```python
from build123d import *

# Parameters (mm, degrees)
SKETCH1_R           = 6.35
SKETCH1_R_2         = 3.175
BOSS_EXTRUDE1_DEPTH = 3.175
SKETCH1_3_R         = 6.35
BOSS_EXTRUDE2_DEPTH = 4.7625
FILLET1_R           = 6.35
SKETCH4_W           = 50.8
SKETCH4_H           = 4.7625
BOSS_EXTRUDE3_DEPTH = 40
SKETCH5_W           = 50.8
SKETCH5_H           = 3.175
BOSS_EXTRUDE4_DEPTH = 88.9
FILLET2_R           = 3.175
SKETCH11_W          = 25.527
SKETCH11_H          = 76.327
CUT_EXTRUDE2_DEPTH  = 125.625465933
SKETCH12_W          = 2.369732381
SKETCH12_H          = 76.327
SKETCH12_W_2        = 2.555200435
BOSS_EXTRUDE5_DEPTH = 1
CUT_EXTRUDE3_DEPTH  = 125.625465933


with BuildPart() as part:
    # Sketch1 → Boss-Extrude1 (new body)
    with BuildSketch(Plane(origin=(0, 0, 0), x_dir=(1, 0, 0), z_dir=(0, 1, 0))):
        with Locations(Location((0, 0, 0), (0, 0, 270))):
            Circle(SKETCH1_R)
        with Locations(Location((0, 0, 0), (0, 0, 270))):
            Circle(SKETCH1_R_2, mode=Mode.SUBTRACT)
    extrude(amount=BOSS_EXTRUDE1_DEPTH)

    # Sketch1_3 → Boss-Extrude2 (add)
    with BuildSketch(Plane(origin=(0, 0, 0), x_dir=(1, 0, 0), z_dir=(0, 1, 0))):
        Polygon((-12.7, -9.525), (-12.7, 0), (-12.7, 22.232248258), (12.7, 22.232248258), (12.7, 0), (12.7, -9.525), align=None)
        with Locations(Location((0, 0, 0), (0, 0, 90))):
            Circle(SKETCH1_3_R, mode=Mode.SUBTRACT)
    extrude(amount=BOSS_EXTRUDE2_DEPTH)

    # Mirror1: part across plane


with BuildPart() as part_1:
    add(part.part)
    add(part.part.mirror(Plane(origin=(12.7, 0, 0), x_dir=(0, 0, 1), z_dir=(1, 0, 0))))

    # Fillet1
    fillet1_edges = [part_1.edges().sort_by_distance(p)[0] for p in [
        (38.1, 2.38125, 9.525),
        (-12.7, 2.38125, 9.525),
    ]]
    fillet(fillet1_edges, radius=FILLET1_R)

    # Sketch4 → Boss-Extrude3 (add)
    with BuildSketch(Plane.XZ):
        with Locations((12.7, -19.850998258)):
            Rectangle(SKETCH4_W, SKETCH4_H)
    extrude(amount=BOSS_EXTRUDE3_DEPTH)

    # Sketch5 → Boss-Extrude4 (add)
    with BuildSketch(Plane(origin=(0, 0, -22.232248258), x_dir=(-1, 0, 0), z_dir=(0, 0, -1))):
        with Locations((-12.7, -38.4125)):
            Rectangle(SKETCH5_W, SKETCH5_H)
    extrude(amount=BOSS_EXTRUDE4_DEPTH)

    # Fillet2
    fillet2_edges = [part_1.edges().sort_by_distance(p)[0] for p in [
        (38.1, -38.4125, -111.132248258),
        (-12.7, -38.4125, -111.132248258),
    ]]
    fillet(fillet2_edges, radius=FILLET2_R)

    # Sketch11 → Cut-Extrude2 (cut, through all)
    with BuildSketch(Plane(origin=(0, -36.825, 0), x_dir=(1, 0, 0), z_dir=(0, 1, 0))):
        with Locations((12.6365, 60.395748258)):
            Rectangle(SKETCH11_W, SKETCH11_H)
    extrude(amount=-CUT_EXTRUDE2_DEPTH, mode=Mode.SUBTRACT)

    # Sketch12 → Boss-Extrude5 (add)
    with BuildSketch(Plane.XZ.offset(40)):
        with Locations((1.05786619, -60.395748258)):
            Rectangle(SKETCH12_W, SKETCH12_H)
        with Locations((24.122399783, -60.395748258)):
            Rectangle(SKETCH12_W_2, SKETCH12_H)
    extrude(amount=-BOSS_EXTRUDE5_DEPTH)

    # Sketch14 → Cut-Extrude3 (cut, through all)
    with BuildSketch(Plane(origin=(0, -36.825, 0), x_dir=(1, 0, 0), z_dir=(0, 1, 0))):
        with BuildLine():
            Line((0.534999946, 104.782248258), (0.534999946, 111.132248258))
            Line((0.534999946, 111.132248258), (24.664999946, 111.132248258))
            Line((24.664999946, 111.132248258), (24.664999946, 104.782248258))
            ThreePointArc((24.664999946, 104.782248258), (24.201028616, 101.468585813), (22.844799565, 98.409783604))
            Line((22.844799565, 98.409783604), (22.844799565, 98.559248258))
            Line((22.844799565, 98.559248258), (2.242732381, 98.559248258))
            Line((2.242732381, 98.559248258), (2.242732381, 98.594257179))
            ThreePointArc((2.242732381, 98.594257179), (0.96976654, 101.572591591), (0.534999946, 104.782248258))
        make_face()
    extrude(amount=-CUT_EXTRUDE3_DEPTH, mode=Mode.SUBTRACT)


solid = part_1.part
```
Here's how the part is built. I have some questions about the finished solid (model axes, mm). A direction names the side the tool comes from. Give positions to 0.01 mm unless a question says otherwise; leave off trailing zeros. Write each loop counter-clockwise with the first axis right and the second up, starting at its lowest first coordinate (ties: lowest second). Pieces come first, ordered by that corner, then holes. Notation, with made-up numbers: M -28,21 L 22,21 A13 cw 22,38 Z; hole C 36.5,64.25 d11. An arc over 180 degrees is marked long. Put each result on its own line as item: value. Start each with the question number.
Item 1: If we section it at A-A, the plane z = -53: Write out the boundary of the cut face in (x, y) (3 decimals), then the cut area to 3 significant figures.
Item 2: On a 3-axis mill with a long thin cutter (end or side, diameter ignored), from which of +Z, -Z, +X, -X, +Y, -Y can I reach the whole of each face in a straight line? I mean faces 4 (the flat face through (24, -39, -60)), 5 (the cylindrical face through (-10.889, 2.415, 7.615)), 6 (the flat face through (0.535, -38, -108)). Say none if no direction works.
Item 3: If we section it at D-D, the plane y = -20: Write out the boundary of the cut face in (x, z), then the cut area to 3 significant figures.
Item 4: Thinking about a two-plate mould opening in X: for faces 1 (the flat face through (-12.7, -38, -40)), 2 (the flat face through (-7, -36.825, -66)), 3 (the flat face through (-0.127, -38, -60)), which applies, +X half, -X half, draft (parallel to the pull), parting line (faces both ways), or undercut?
Item 5: I need wall thicknesses on L1, parallel to X at y = 2.35, z = 0 (3 decimals); L2, parallel to Z at x = 25.4, y = 1.15 (3 decimals); L3, parallel to Z at x = 0, y = 4 (3 decimals). Which ranges of each line are inside material? Lowest first, please. Write a range as from..to.
Item 6: Will these pins go through, and if not, where does the flat tip stop? pin 1 (1.5 mm diameter, centred on x = 14, y = -10.5, fed in from +Z); pin 2 (14.5 mm diameter, centred on x = 0, z = 0, fed in from +Y); pin 3 (8 mm diameter, centred on x = 14.5, z = 2.5, fed in from -Y); pin 4 (16.5 mm diameter, centred on x = 27.5, z = -78.5, fed in from +Y) (3 decimals).
Item 7: If we section it at C-C, the plane x = 13: Write out the boundary of the cut face in (y, z) (1 decimal).
Item 8: If we section it at B-B, the plane z = 0: Count the separate pieces of the cut face and the enclosed holes in it, then the cut area to 3 significant figures.
Values:
1. outline: M -12.7,-40 L 2.243,-40 L 2.243,-39 L -0.127,-39 L -0.127,-36.825 L -12.7,-36.825 Z; M 22.845,-40 L 38.1,-40 L 38.1,-36.825 L 25.4,-36.825 L 25.4,-39 L 22.845,-39 Z
1. area: 85.2 mm²
2. face 4: +Y
2. face 5: +Z, -X, +Y, -Y
2. face 6: -Z, +Y, -Y
3. outline: M -12.7,-22.23 L 38.1,-22.23 L 38.1,-17.47 L -12.7,-17.47 Z
3. area: 242 mm²
4. face 1: -X half
4. face 2: draft
4. face 3: undercut
5. L1: -12.7..-3.175, 3.175..22.225, 28.575..38.1
5. L2: -22.232..-3.175, 3.175..9.525
5. L3: -22.232..-6.35, 6.35..9.525
6. pin 1: z = -17.47
6. pin 2: y = 4.76
6. pin 3: y = 0
6. pin 4: y = -36.825
7. outline: M -40,-22.2 L 4.8,-22.2 L 4.8,9.5 L 0,9.5 L 0,-17.5 L -40,-17.5 Z
8. separate pieces: 3
8. enclosed holes: 0
8. area: 161 mm²
